Read the model definition and answer for the solid it produces. Units are mm, in the model's axes. Give positions to 0.01 mm unless a question says otherwise; leave off trailing zeros. Order: outer loops, then holes, each group sorted by start corner. A loop starts at its lowest first (then second) coordinate and runs counter-clockwise, first axis right, second up. Notation, with made-up numbers: M -28,35.5 L 17,35.5 A21 ccw 17,62.5 Z; hole C 31,28 d9. An arc over 180 degrees is marked long. One line per item, written item: value. Start each with the question number.
from build123d import *

# Parameters (mm, degrees)
F1_DEPTH       = 2020
F3_D           = 4.5
F3_CBORE_D     = 7.5
F3_CBORE_DEPTH = 6


with BuildPart() as f1:
    # F0 (on Right) → F1 (new body)
    with BuildSketch(Plane.YZ):
        with BuildLine():
            Line((-2.5, 0.5), (0, 0.5))
            Line((0, 0.5), (2.5, 0.5))
            Line((2.5, 0.5), (3, 0))
            Line((3, 0), (7, 0))
            Line((7, 0), (7.5, 0.5))
            Line((7.5, 0.5), (7.5, 3.3))
            Line((7.5, 3.3), (5.37868, 5.42132))
            Line((5.37868, 5.42132), (5.37868, 7.257359))
            Line((5.37868, 7.257359), (5.503925, 7.382605))
            ThreePointArc((5.503925, 7.382605), (6.085786, 8.671573), (7.374754, 9.253434))
            Line((7.374754, 9.253434), (7.5, 9.37868))
            Line((7.5, 9.37868), (7.5, 10.87868))
            Line((7.5, 10.87868), (7.374754, 11.003925))
            ThreePointArc((7.374754, 11.003925), (6.085786, 11.585786), (5.503925, 12.874754))
            Line((5.503925, 12.874754), (5.37868, 13))
            Line((5.37868, 13), (0, 13))
            Line((0, 13), (-5.37868, 13))
            Line((-5.37868, 13), (-5.503925, 12.874754))
            ThreePointArc((-5.503925, 12.874754), (-6.085786, 11.585786), (-7.374754, 11.003925))
            Line((-7.374754, 11.003925), (-7.5, 10.87868))
            Line((-7.5, 10.87868), (-7.5, 9.37868))
            Line((-7.5, 9.37868), (-7.374754, 9.253434))
            ThreePointArc((-7.374754, 9.253434), (-6.085786, 8.671573), (-5.503925, 7.382605))
            Line((-5.503925, 7.382605), (-5.37868, 7.257359))
            Line((-5.37868, 7.257359), (-5.37868, 5.42132))
            Line((-5.37868, 5.42132), (-7.5, 3.3))
            Line((-7.5, 3.3), (-7.5, 0.5))
            Line((-7.5, 0.5), (-7, 0))
            Line((-7, 0), (-3, 0))
            Line((-3, 0), (-2.5, 0.5))
        make_face()
    extrude(amount=F1_DEPTH)

    # F3 (through all)
    with Locations(Plane.XY.offset(13)):
        with Locations((20, 0), (80, 0), (140, 0), (200, 0), (260, 0), (320, 0), (380, 0), (440, 0), (500, 0), (560, 0), (620, 0), (680, 0), (740, 0), (800, 0), (860, 0), (920, 0), (980, 0), (1040, 0), (1100, 0), (1160, 0), (1220, 0), (1280, 0), (1340, 0), (1400, 0), (1460, 0), (1520, 0), (1580, 0), (1640, 0), (1700, 0), (1760, 0), (1820, 0), (1880, 0), (1940, 0), (2000, 0)):
            CounterBoreHole(F3_D / 2, F3_CBORE_D / 2, F3_CBORE_DEPTH)


solid = f1.part
Q1. Each of these flat-tipped pins is pushed along its axis until it touches: pin 1 (6 mm diameter, centred on x = 1820, y = 0, fed in from +Z); pin 2 (2 mm diameter, centred on x = 505, z = 6, fed in from -Y). Where does it stop, or does it pass through?
Q2. Consider probe 1 along Y at (x, z) = (1100, 3.75); probe 2 along Z at (x, y) = (1664, -6.75); probe 3 along Y at (x, z) = (140, 4). Determine where each line is inside the solid, lowest interval first.
Q3. Find section A-A, the plane x = 822.5. Give the vertices of the cut face in (y, z).
Evaluation:
1. pin 1: z = 7
1. pin 2: y = -5.8
2. probe 1: -7.05 to -2.25, 2.25 to 7.05
2. probe 2: 0 to 4.05, 9.11 to 11.15
2. probe 3: -6.8 to -2.25, 2.25 to 6.8
3. outline: M -7.5,0.5 L -7,0 L -3,0 L -2.5,0.5 L 2.5,0.5 L 3,0 L 7,0 L 7.5,0.5 L 7.5,3.3 L 5.38,5.42 L 5.38,7.26 L 5.5,7.38 A2 cw 7.37,9.25 L 7.5,9.38 L 7.5,10.88 L 7.37,11 A2 cw 5.5,12.87 L 5.38,13 L -5.38,13 L -5.5,12.87 A2 cw -7.37,11 L -7.5,10.88 L -7.5,9.38 L -7.37,9.25 A2 cw -5.5,7.38 L -5.38,7.26 L -5.38,5.42 L -7.5,3.3 Z
